Geometry: see drawing. Coordinates: mm, zero at the bounding-box minimum. Round coordinates to 2 decimals unless told otherwise and drop trailing zeros. Order: outer loops, then holes, each group sorted by start corner. A loop starts at its lowest first (then second) coordinate and runs counter-clockwise, first axis right, second up. Notation, with made-up numbers: (36.25, 0) -> (76.25, 0) arc R22 ccw to (76.25, 17) -> close; hole circle Ø10 at (11.25, 56). An arc over 180 degrees is marked (long way). Use a Markdown table: item, result.
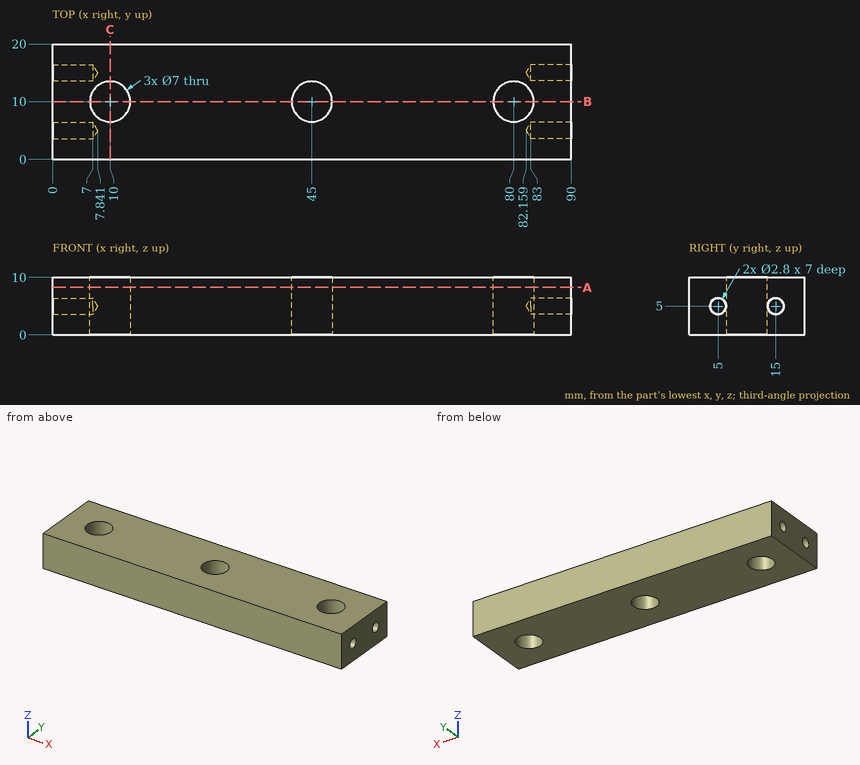
1) Contact query for flat-ended pins moving along their axis: P1, Ø5.5, axis at x = 45, y = 10, coming from the +Z side; P2, Ø1.7, axis at y = 5, z = 5, coming from the -X side; P3, Ø2, axis at y = 15, z = 5, coming from the -X side. Output: stop coordinate, or through.
Answer key:
| item | result |
|---|---|
| P1 | passes through |
| P2 | stops at x = 7.33 |
| P3 | stops at x = 7.24 |
2) Cut plane B-B on y = 10. Return loops of the section in (x, z), and give its area (3 significant figures).
Answer key:
| item | result |
|---|---|
| outline | (0, 0) -> (6.5, 0) -> (6.5, 10) -> (0, 10) -> close; (13.5, 0) -> (41.5, 0) -> (41.5, 10) -> (13.5, 10) -> close; (48.5, 0) -> (76.5, 0) -> (76.5, 10) -> (48.5, 10) -> close; (83.5, 0) -> (90, 0) -> (90, 10) -> (83.5, 10) -> close |
| area | 690 mm^2 |
3) Cut plane A-A on z = 8.25. Return loops of the section in (x, y).
Answer key:
| item | result |
|---|---|
| outline | (0, 0) -> (90, 0) -> (90, 20) -> (0, 20) -> close; hole circle Ø7 at (10, 10); hole circle Ø7 at (45, 10); hole circle Ø7 at (80, 10) |
4) Cut plane C-C on x = 10. Return loops of the section in (y, z).
Answer key:
| item | result |
|---|---|
| outline | (0, 0) -> (6.5, 0) -> (6.5, 10) -> (0, 10) -> close; (13.5, 0) -> (20, 0) -> (20, 10) -> (13.5, 10) -> close |
5) Ray query, probe 1 along Y at (x, z) = (5.25, 5); probe 2 along X at (y, z) = (11.25, 9.25); probe 3 along Y at (x, z) = (80, 6.5). Return the intervals inside material, ascending.
Answer key:
| item | result |
|---|---|
| probe 1 | y = 0 to 3.6, 6.4 to 13.6, 16.4 to 20 |
| probe 2 | x = 0 to 6.73, 13.27 to 41.73, 48.27 to 76.73, 83.27 to 90 |
| probe 3 | y = 0 to 6.5, 13.5 to 20 |
